```python
from build123d import *

# Parameters (mm, degrees)
SKETCH_1_R                   = 38
EXTRUDE_1_DEPTH              = 20
SKETCH_2_R                   = 27.5
EXTRUDE_2_DEPTH              = 5.5
HOLE_WIZARD_M5_1_D           = 4.2
HOLE_WIZARD_M5_1_CSINK_D     = 5.05
HOLE_WIZARD_M5_1_CSINK_ANGLE = 90
HOLE_WIZARD_M4_1_D           = 3.3
HOLE_WIZARD_M4_1_DEPTH       = 10.1
HOLE_WIZARD_M4_1_CSINK_D     = 4.05
HOLE_WIZARD_M4_1_CSINK_ANGLE = 90
HOLE_WIZARD_M4_1_TIP         = 0.991420021
FILLET_1_R                   = 0.25


with BuildPart() as part:
    # 草图1 → 凸台-拉伸1 (new, symmetric)
    with BuildSketch(Plane.XY):
        Circle(SKETCH_1_R)
    extrude(amount=EXTRUDE_1_DEPTH, both=True)

    # 草图2 → 凸台-拉伸2 (add)
    with BuildSketch(Plane.XY.offset(20)):
        Circle(SKETCH_2_R)
    extrude(amount=EXTRUDE_2_DEPTH)

    # M5 螺纹孔1 (through all)
    with Locations(Plane(origin=(0, 33, -20), x_dir=(-1, 0, 0), z_dir=(0, 0, -1))):
        with Locations((0, 0), (23.334523779, -9.665476221), (33, -33), (23.334523779, -56.334523779), (0, -66), (-23.334523779, -56.334523779), (-33, -33), (-23.334523779, -9.665476221)):
            CounterSinkHole(HOLE_WIZARD_M5_1_D / 2, HOLE_WIZARD_M5_1_CSINK_D / 2, counter_sink_angle=HOLE_WIZARD_M5_1_CSINK_ANGLE)

    # M4 螺纹孔1
    with Locations(Plane(origin=(0, 22.5, 25.5), x_dir=(1, 0, 0), z_dir=(0, 0, 1))):
        with Locations((0, 0), (19.485571585, -11.25), (19.485571585, -33.75), (0, -45), (-19.485571585, -33.75), (-19.485571585, -11.25)):
            CounterSinkHole(HOLE_WIZARD_M4_1_D / 2, HOLE_WIZARD_M4_1_CSINK_D / 2, depth=HOLE_WIZARD_M4_1_DEPTH, counter_sink_angle=HOLE_WIZARD_M4_1_CSINK_ANGLE)
            with Locations((0, 0, -(HOLE_WIZARD_M4_1_DEPTH + HOLE_WIZARD_M4_1_TIP / 2))):  # 118° drill point
                Cone(0, HOLE_WIZARD_M4_1_D / 2, HOLE_WIZARD_M4_1_TIP, mode=Mode.SUBTRACT)

    # 圆角1
    fillet_1_edges = [part.edges().sort_by_distance(p)[0] for p in [
        (-38, 0, -20),
        (-38, 0, 20),
        (-27.5, 0, 25.5),
    ]]
    fillet(fillet_1_edges, radius=FILLET_1_R)


solid = part.part
```
Here's how the part is built. I have some questions about the finished solid (model axes, mm). A direction names the side the tool comes from. Give positions to 0.01 mm unless a question says otherwise; leave off trailing zeros. Order: outer loops, then holes, each group sorted by start corner. A loop starts at its lowest first (then second) coordinate and runs counter-clockwise, first axis right, second up. Notation, with made-up numbers: M 17.5,-4.5 L 37.5,-4.5 A27 cw 37.5,29.5 Z; hole C 59,-31 d9. An arc over 180 degrees is marked long. Use a Markdown table: item, result. Add a question column.
1. If we mould it in two halves opening along X, with no side actions, what happens to faces 1 (the cylindrical face through (-22.21, -21.56, 0.49)), 2 (the cylindrical face through (17.535, -33.713, 0.276)), 3 (the flat face through (-1, 1, -20)), 4 (the conical face through (19.45, 11.53, 14.58))? For each: +X half, -X half, draft (parallel to the pull), parting line (faces both ways), or undercut.
2. For pin 1 Ø5 at (y, z) = (-7, -7) entering from +X; pin 2 Ø4 at (x, y) = (-24.5, -29) entering from -Z; pin 3 Ø1 at (x, z) = (-3.5, 8.5) entering from -Y; pin 4 Ø4 at (y, z) = (17, 12.5) entering from +X, each with a flat end and sliding along its axis, tell me the tip position at first contact or that it passes through.
3. Suppose I cut it at A-A (y = 0). List the corners of the cut face in (x, z) for me (3 decimals), and give its area (3 significant figures).
4. I need wall thicknesses on probe 1 along Y at (x, z) = (0, 5.5); probe 2 along Y at (x, z) = (0, 23); probe 3 along Z at (x, y) = (4.5, -33.5). Which ranges of each line are inside material? Lowest first, please. Write a range as from..to.
5. On a 3-axis mill with a long thin cutter (end or side, diameter ignored), from which of +Z, -Z, +X, -X, +Y, -Y can I reach the whole of each face in a straight line? I mean faces 5 (the cylindrical face through (-22.37, 21.47, 0.49)), 6 (the cylindrical face through (0.215, 24.136, 20.194)). Say none if no direction works.
Results list:
| question | item | result |
|---|---|---|
| 1 | face 1 | undercut |
| 1 | face 2 | parting line |
| 1 | face 3 | draft |
| 1 | face 4 | undercut |
| 2 | pin 1 | stops at x = 37.73 |
| 2 | pin 2 | stops at z = -20 |
| 2 | pin 3 | stops at y = -37.88 |
| 2 | pin 4 | stops at x = 34.91 |
| 3 | outline | M -38,-19.75 A0.25 ccw -37.75,-20 L -35.525,-20 L -35.1,-19.575 L -35.1,20 L -37.75,20 A0.25 ccw -38,19.75 Z; M -30.9,-19.575 L -30.475,-20 L 30.475,-20 L 30.9,-19.575 L 30.9,20 L 27.5,20 L 27.5,25.25 A0.25 ccw 27.25,25.5 L -27.25,25.5 A0.25 ccw -27.5,25.25 L -27.5,20 L -30.9,20 Z; M 35.1,-19.575 L 35.525,-20 L 37.75,-20 A0.25 ccw 38,-19.75 L 38,19.75 A0.25 ccw 37.75,20 L 35.1,20 Z |
| 3 | area | 3,010 mm² |
| 4 | probe 1 | y = -38..-35.1, -30.9..30.9, 35.1..38 |
| 4 | probe 2 | y = -27.5..-24.15, -20.85..20.85, 24.15..27.5 |
| 4 | probe 3 | z = -20..20 |
| 5 | face 5 | +Z, -Z |
| 5 | face 6 | +Z |
